Autodesk Fusion 360 part; units mm, degrees
sketch "Sketch1" plane through (0, 0, 0) normal (0, 0, 1) x (1, 0, 0)
  line L0 (39, 192) -> (77, 192)
  line L1 (77, 192) -> (77, 186)
  line L2 (39, 186) -> (39, 192)
  line L3 (115, 192) -> (153, 192)
  line L4 (153, 192) -> (153, 186)
  line L5 (115, 186) -> (115, 192)
  line L6 (39, 186) -> (0, 186)
  line L7 (77, 186) -> (115, 186)
  line L8 (153, 186) -> (192, 186)
  line L9 (39, 6) -> (0, 6)
  line L10 (39, 6) -> (39, 0)
  line L11 (39, 0) -> (77, 0)
  line L12 (77, 0) -> (77, 6)
  line L13 (77, 6) -> (115, 6)
  line L14 (115, 6) -> (115, 0)
  line L15 (115, 0) -> (153, 0)
  line L16 (153, 0) -> (153, 6)
  line L17 (153, 192) -> (115, 192)
  line L18 (77, 192) -> (39, 192)
  line L19 (39, 0) -> (77, 0)
  line L20 (115, 0) -> (153, 0)
  line L21 (6, 153) -> (0, 153)
  line L22 (0, 153) -> (0, 186)
  line L23 (6, 39) -> (0, 39)
  line L24 (0, 39) -> (0, 6)
  line L25 (0, 115) -> (6, 115)
  line L26 (6, 77) -> (0, 77)
  line L27 (0, 77) -> (0, 115)
  line L28 (6, 39) -> (6, 77)
  line L29 (6, 115) -> (6, 153)
  line L30 (192, 153) -> (192, 186)
  line L31 (186, 153) -> (192, 153)
  line L32 (186, 115) -> (186, 153)
  line L33 (192, 115) -> (186, 115)
  line L34 (192, 77) -> (192, 115)
  line L35 (186, 77) -> (192, 77)
  line L36 (186, 39) -> (186, 77)
  line L37 (186, 39) -> (192, 39)
  line L38 (192, 39) -> (192, 6)
  line L39 (192, 153) -> (192, 186)
  line L40 (192, 6) -> (192, 39)
  line L41 (192, 77) -> (192, 115)
  line L42 (0, 39) -> (0, 6)
  line L43 (0, 186) -> (0, 153)
  line L44 (0, 115) -> (0, 77)
  line L45 (153, 6) -> (192, 6)
  line L46 (5.915, 152.915) -> (-0.085, 152.915)
  line L47 (-0.085, 186.085) -> (-0.085, 152.915)
  line L48 (38.915, 186.085) -> (-0.085, 186.085)
  line L49 (38.915, 186.085) -> (38.915, 192.085)
  line L50 (77.085, 192.085) -> (38.915, 192.085)
  line L51 (77.085, 192.085) -> (77.085, 186.085)
  line L52 (77.085, 186.085) -> (114.915, 186.085)
  line L53 (114.915, 186.085) -> (114.915, 192.085)
  line L54 (114.915, 192.085) -> (153.085, 192.085)
  line L55 (153.085, 192.085) -> (153.085, 186.085)
  line L56 (153.085, 186.085) -> (192.085, 186.085)
  line L57 (192.085, 152.915) -> (192.085, 186.085)
  line L58 (186.085, 152.915) -> (192.085, 152.915)
  line L59 (186.085, 115.085) -> (186.085, 152.915)
  line L60 (192.085, 115.085) -> (186.085, 115.085)
  line L61 (192.085, 76.915) -> (192.085, 115.085)
  line L62 (186.085, 76.915) -> (192.085, 76.915)
  line L63 (186.085, 39.085) -> (186.085, 76.915)
  line L64 (186.085, 39.085) -> (192.085, 39.085)
  line L65 (192.085, 39.085) -> (192.085, 5.915)
  line L66 (153.085, 5.915) -> (192.085, 5.915)
  line L67 (153.085, -0.085) -> (153.085, 5.915)
  line L68 (114.915, -0.085) -> (153.085, -0.085)
  line L69 (114.915, 5.915) -> (114.915, -0.085)
  line L70 (77.085, 5.915) -> (114.915, 5.915)
  line L71 (77.085, -0.085) -> (77.085, 5.915)
  line L72 (38.915, -0.085) -> (77.085, -0.085)
  line L73 (38.915, 5.915) -> (38.915, -0.085)
  line L74 (38.915, 5.915) -> (-0.085, 5.915)
  line L75 (-0.085, 39.085) -> (-0.085, 5.915)
  line L76 (5.915, 39.085) -> (-0.085, 39.085)
  line L77 (5.915, 39.085) -> (5.915, 76.915)
  line L78 (5.915, 76.915) -> (-0.085, 76.915)
  line L79 (-0.085, 115.085) -> (-0.085, 76.915)
  line L80 (-0.085, 115.085) -> (5.915, 115.085)
  line L81 (5.915, 115.085) -> (5.915, 152.915)
  dimension "d3" = 38
  dimension "d4" = 6
  dimension "d5" = 38
  dimension "d6" = 6
  dimension "d7" = 39
  dimension "d8" = 39
  dimension "d10" = 33
  dimension "d12" = 33
  dimension "d13" = 6
  dimension "d14" = 38
  dimension "d15" = 38
  dimension "d16" = 38
  dimension "d19" = 0.085
extrude "Extrude1" add sketch "Sketch1" along normal blind 6 contours L0 L1 L2 L3 L4 L5 L6 L7 L8 L9 L10 L11 L12 L13 L14 L15 L16 L17 L18 L19 L20 L21 L22 L23 L24 L25 L26 L27 L28 L29 L30 L31 L32 L33 L34 L35 L36 L37 L38 L39 L40 L41 L42 L43 L44 L45
extrude "Extrude2" cut 2 faces at (51.6667, 192, 4) (127.6667, 192, 4) along direction (0, -1, 0) blind 1
extrude "Extrude3" cut 3 faces at (192, 28, 2) (192, 89.6667, 4) (192, 164, 4) along direction (-1, 0, 0) blind 1
extrude "Extrude4" cut 2 faces at (51.6667, 0, 4) (127.6667, 0, 4) along direction (0, 1, 0) blind 1
extrude "Extrude5" cut 3 faces at (0, 164, 4) (0, 89.6667, 4) (0, 28, 2) along direction (1, 0, 0) blind 1
The listing builds one solid part. Answer for the finished solid, in the listing's coordinates (mm). A direction names the side the tool comes from. Coordinates: 2 decimals unless noted, no trailing zeros. Write each loop counter-clockwise with the first axis right and the second up, starting at its lowest first coordinate (ties: lowest second). Pieces come first, ordered by that corner, then holes. Notation, with made-up numbers: (72, 69.5) -> (80, 69.5) arc R36 cw to (80, 108.5) -> close; hole circle Ø2 at (6, 30.25). An arc over 180 degrees is marked (long way). One line per question, with ' | ' between items.
1. Section A-A (y = 66.5) is taken. Determine the outline of the cut face in (x, z), and give its area (3 significant figures).
Verdict:
outline: (6, 0) -> (186, 0) -> (186, 6) -> (6, 6) -> close | area: 1,080 mm^2
2. Given pin 1 Ø1 at (x, z) = (169.5, 1) entering from +Y; pin 2 Ø3 at (y, z) = (133, 3) entering from -X; pin 3 Ø1.5 at (y, z) = (4, 4) entering from -X, each flat-ended and moving along its own axis, determine where each tip first touches the part or whether it passes through.
Verdict:
pin 1: stops at y = 186 | pin 2: stops at x = 6 | pin 3: stops at x = 39
3. Which of the six approach directions +Z, -Z, +X, -X, +Y, -Y give full straight-line access (tool end or side, diameter ignored) to faces 4 (the flat face through (153, 3, 3)), 5 (the flat face through (4, 77, 3)), 6 (the flat face through (186, 58, 3)), 7 (the flat face through (96, 6, 3))?
Verdict:
face 4: +Z, -Z, +X, -Y | face 5: +Z, -Z, -X | face 6: +Z, -Z, +X | face 7: +Z, -Z, -Y
4. For a pull along X with two mould halves and no side action, classify faces 1 (the flat face through (191, 23, 3)), 2 (the flat face through (6, 58, 3)), 3 (the flat face through (115, 188, 3)) as released by +X, released by -X, zero draft, split by the parting line, or undercut.
Verdict:
face 1: released by +X | face 2: released by -X | face 3: undercut
5. A straight line is drawn through the part: line 1 (X direction, y = 126, z = 1.8). Find the intervals that lie inside material, in ascending order.
Verdict:
line 1: x = 6 to 186
